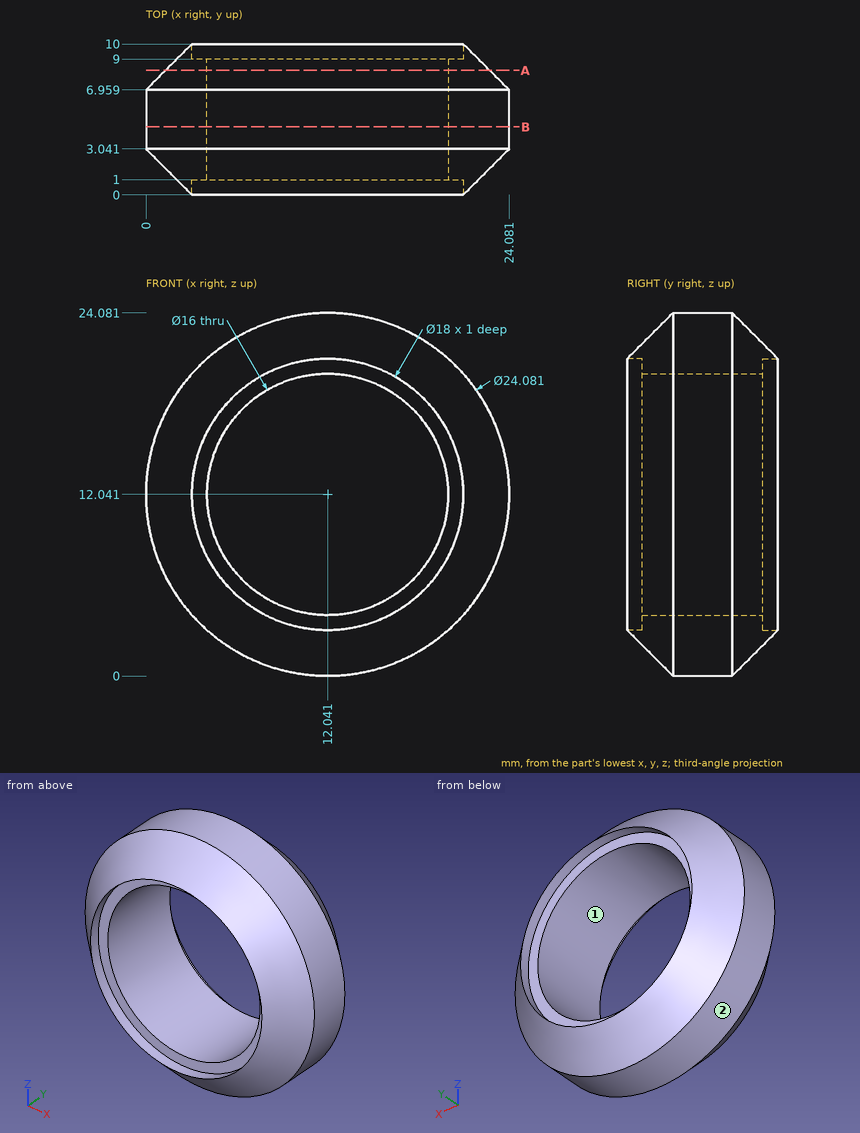
Check sheet for the drawn part. Datum: minimum x, y, z corner. Units: mm. Round coordinates to 2 decimals unless told otherwise and drop trailing zeros. Order: outer loops, then holes, each group sorted by start corner. A loop starts at its lowest first (then second) coordinate and runs counter-clockwise, first axis right, second up.
1) Section check A-A (y = 8.25). Record the boundary of the cut face in (x, z), and give its area (3 significant figures).
2) Section check B-B (y = 4.5). Record the boundary of the cut face in (x, z).
3) Go/stop test with flat-tipped pins: pin 1 Ø5 at (y, z) = (1, 6) entering from +X; pin 2 Ø1 at (x, y) = (9.5, 8.5) entering from -Z (1 decimal); pin 3 Ø10 at (x, z) = (6, 15) entering from +Y. Record where each tip stops, or that it passes through.
4) Scan lines: line 1 (X direction, y = 4, z = 12); line 2 (Y direction, x = 17, z = 5); line 3 (X direction, y = 3, z = 10.25) (1 decimal). Record each from-to range of solid material in increasing order.
5) Mould release check, pull along X, two halves, no side actions. Record for the marked faces 1 and 2: +X half, -X half, draft (parallel to the pull), parting line (faces both ways), or undercut.
Result:
1. outline: circle Ø21.5 at (12.04, 12.04); hole circle Ø16 at (12.04, 12.04)
1. area: 162 mm2
2. outline: circle Ø24.08 at (12.04, 12.04); hole circle Ø16 at (12.04, 12.04)
3. pin 1: stops at x = 23.17
3. pin 2: stops at z = 1.3
3. pin 3: stops at y = 10
4. line 1: x = 0 to 4.04, 20.04 to 24.08
4. line 2: y = 1 to 9
4. line 3: x = 0.2 to 4.2, 19.8 to 23.9
5. face 1: undercut
5. face 2: parting line
